CAD build for the part. Positions are in the model's coordinates, mm. A direction names the side the tool comes from. Round coordinates to 2 decimals unless told otherwise and drop trailing zeros. Order: outer loops, then holes, each group sorted by start corner. A loop starts at its lowest first (then second) coordinate and runs counter-clockwise, first axis right, second up. Notation, with made-up numbers: M 9.25,56.5 L 40.25,56.5 A14 cw 40.25,60.5 Z; hole C 50,6 d6. An arc over 180 degrees is marked long. Answer as a JSON object with one key per item and string values.
```python
from build123d import *

# Parameters (mm, degrees)
F0_W     = 22.86
F0_H     = 10.541
F0_W_2   = 17.78
F0_H_2   = 4.064
F1_DEPTH = 0.762
F2_W     = 19.304
F2_H     = 7.62
F2_W_2   = 17.78
F2_H_2   = 4.064
F3_DEPTH = 10.5918


with BuildPart() as f1:
    # F0 (on Front) → F1 (new body)
    with BuildSketch(Plane.XZ):
        Rectangle(F0_W, F0_H)
        Rectangle(F0_W_2, F0_H_2, mode=Mode.SUBTRACT)
    extrude(amount=F1_DEPTH)

    # F2 (on face) → F3 (join)
    with BuildSketch(Plane.XZ.offset(0.762)):
        Rectangle(F2_W, F2_H)
        Rectangle(F2_W_2, F2_H_2, mode=Mode.SUBTRACT)
    extrude(amount=F3_DEPTH)


solid = f1.part
```
Item 1: Saw through at A-A on x = 8.25. List the corners of the cut face in (y, z), and give its area (3 significant figures).
Worked answers:
{"outline": "M -11.35,-3.81 L -0.76,-3.81 L -0.76,-5.27 L 0,-5.27 L 0,-2.03 L -11.35,-2.03 Z; M -11.35,2.03 L 0,2.03 L 0,5.27 L -0.76,5.27 L -0.76,3.81 L -11.35,3.81 Z", "area": "42.6 mm2"}
Item 2: Drop flat-ended pins along their axis: pin 1 Ø5.5 at (x, y) = (4.5, -4) entering from -Z; pin 2 Ø6 at (y, z) = (-8.5, 0.5) entering from +X; pin 3 Ø3.5 at (y, z) = (-4.5, 0.5) entering from -X. Give the stop position or say it passes through.
Worked answers:
{"pin 1": "stops at z = -3.81", "pin 2": "stops at x = 9.65", "pin 3": "stops at x = -9.65"}
Item 3: 3-axis set-ups, long thin cutter, end or side, ignore diameter. For faces 5 (the flat face through (-8.89, -6, 0)), 6 (the flat face through (9.652, -6, 0)), 7 (the flat face through (-9.652, -6, 0)), 8 (the flat face through (0, -11.354, 3)): which of +Z, -Z, +X, -X, +Y, -Y reach the whole face in a straight line?
Worked answers:
{"face 5": "+Y, -Y", "face 6": "+Z, -Z, +X, -Y", "face 7": "+Z, -Z, -X, -Y", "face 8": "+Z, -Z, +X, -X, -Y"}
Item 4: Wall check: line 1 along Z through (x, y) = (-6, -9.75); line 2 along X through (y, z) = (-4.5, 2); line 3 along Y through (x, z) = (-6.5, -4.5). Give the ranges that are in metal, low to high. Write a range as [from, to].
Worked answers:
{"line 1": "z = [-3.81, -2.03], [2.03, 3.81]", "line 2": "x = [-9.65, -8.89], [8.89, 9.65]", "line 3": "y = [-0.76, 0]"}
Item 5: Saw through at C-C on z = -1.25. List the corners of the cut face in (x, y).
Worked answers:
{"outline": "M -11.43,-0.76 L -9.65,-0.76 L -9.65,-11.35 L -8.89,-11.35 L -8.89,0 L -11.43,0 Z; M 8.89,-11.35 L 9.65,-11.35 L 9.65,-0.76 L 11.43,-0.76 L 11.43,0 L 8.89,0 Z"}
Item 6: Saw through at B-B on y = -7.25. List the corners of the cut face in (x, z).
Worked answers:
{"outline": "M -9.65,-3.81 L 9.65,-3.81 L 9.65,3.81 L -9.65,3.81 Z; hole M -8.89,-2.03 L 8.89,-2.03 L 8.89,2.03 L -8.89,2.03 Z"}
Item 7: Two-plate mould, pull along Z, no slides. Class faces 1 (the flat face through (0, -0.762, -5)), 2 (the flat face through (0, -6, -2.032)), 3 (the flat face through (0, -6, -3.81)), 4 (the flat face through (0, -6, 3.81)): released by +Z, released by -Z, zero draft, split by the parting line, or undercut.
Worked answers:
{"face 1": "zero draft", "face 2": "undercut", "face 3": "released by -Z", "face 4": "released by +Z"}
Item 8: Saw through at D-D on z = 3.5. List the corners of the cut face in (x, y), and give its area (3 significant figures).
Worked answers:
{"outline": "M -11.43,-0.76 L -9.65,-0.76 L -9.65,-11.35 L 9.65,-11.35 L 9.65,-0.76 L 11.43,-0.76 L 11.43,0 L -11.43,0 Z", "area": "222 mm2"}
